Could you check a few things on this model? Use its own coordinates, in mm. Coordinates: 2 decimals unless noted, no trailing zeros. Loops run counter-clockwise (first coordinate to the right, second up) from the corner with the lowest first, then second, coordinate; pieces in that order, holes last. Notation, with made-up numbers: (57.25, 55.25) - (90.25, 55.25) arc R29 ccw to (90.25, 83.25) - close; hole circle Ø10 at (-29.75, 55). An arc over 180 degrees is marked (long way). One line per question, with ' | ' between items. Start each with the question number.
1. Please list where these lines run through material, in increasing order: L1, parallel to Y at x = -16.5, z = 0.25; L2, parallel to X at y = 40.5, z = 0; L3, parallel to Y at x = -9.5, z = 0.45. Write a range as [from, to].
2. I want a section at A-A, the plane x = 0. Write out the boundary of the cut face in (y, z), then the cut area to 3 significant figures.
3. I want a section at C-C, the plane z = -0.1. Count the separate pieces of the cut face and the enclosed holes in it, then the cut area to 3 significant figures.
4. I'm going to push a flat-ended pin straight in: P1, Ø0.5, axis at x = -40.5, z = -0.5, coming from the +Y side. Where does the tip first touch, or does it pass through?
5. I want a section at B-B, the plane x = -16.5. Write out the boundary of the cut face in (y, z), then the cut area to 3 significant figures.
from build123d import *

# Parameters (mm, degrees)
SKETCH2_W            = 82.5
SKETCH2_H            = 99
SKETCH2_R            = 0.8
SKETCH2_R_2          = 1.5
PCB_EXTRUDE_DEPTH    = 0.8
CORNER_FILLETS_R     = 1
SKETCH4_R            = 1.5
SOLAR_HOLES_DEPTH    = 65.454421881
SOLAR_HOLE_FILLETS_R = 0.5
M2_CLEARANCE_HOLES_D = 2.6
SKETCH10_W           = 1.75
SKETCH10_H           = 2.6
CUT_EXTRUDE2_DEPTH   = 65.454421881


with BuildPart() as part:
    # Sketch2 → pcb extrude (new, symmetric)
    with BuildSketch(Plane.XY):
        Rectangle(SKETCH2_W, SKETCH2_H)
        with Locations((0, 46.95)):
            Circle(SKETCH2_R, mode=Mode.SUBTRACT)
        with Locations((-39.5, -30.25)):
            Circle(SKETCH2_R, mode=Mode.SUBTRACT)
        with Locations((-39.5, -0.25)):
            Circle(SKETCH2_R, mode=Mode.SUBTRACT)
        with Locations((-39.5, 29.75)):
            Circle(SKETCH2_R, mode=Mode.SUBTRACT)
        with Locations((39.5, -30.25)):
            Circle(SKETCH2_R, mode=Mode.SUBTRACT)
        with Locations((39.5, -0.25)):
            Circle(SKETCH2_R, mode=Mode.SUBTRACT)
        with Locations((39.5, 29.75)):
            Circle(SKETCH2_R, mode=Mode.SUBTRACT)
        with Locations((0, -46.95)):
            Circle(SKETCH2_R_2, mode=Mode.SUBTRACT)
        with Locations((-16.5, 20)):
            Circle(SKETCH2_R, mode=Mode.SUBTRACT)
        with Locations((16.5, 20)):
            Circle(SKETCH2_R, mode=Mode.SUBTRACT)
        with Locations((-16.5, -20)):
            Circle(SKETCH2_R, mode=Mode.SUBTRACT)
        with Locations((16.5, -20)):
            Circle(SKETCH2_R, mode=Mode.SUBTRACT)
    extrude(amount=PCB_EXTRUDE_DEPTH, both=True)

    # corner fillets
    corner_fillets_edges = [part.edges().sort_by_distance(p)[0] for p in [
        (41.25, 49.5, 0),
        (41.25, -49.5, 0),
        (-41.25, -49.5, 0),
        (-41.25, 49.5, 0),
    ]]
    fillet(corner_fillets_edges, radius=CORNER_FILLETS_R)

    # Sketch4 → solar holes (cut, through all)
    with BuildSketch(Plane.XY.offset(0.8)):
        with Locations((0, 46.95)):
            Circle(SKETCH4_R)
        with BuildLine():
            Line((6.7, 39.35), (-6.7, 39.35))
            Line((-6.7, 39.35), (-6.7, 46.65))
            Line((-6.7, 46.65), (-9.5, 46.65))
            ThreePointArc((-9.5, 46.65), (-10, 47.15), (-9.5, 47.65))
            Line((-9.5, 47.65), (-3, 47.65))
            Line((-3, 47.65), (-3, 45.05))
            Line((-3, 45.05), (3, 45.05))
            Line((3, 45.05), (3, 47.65))
            Line((3, 47.65), (9.5, 47.65))
            ThreePointArc((9.5, 47.65), (10, 47.15), (9.5, 46.65))
            Line((9.5, 46.65), (6.7, 46.65))
            Line((6.7, 46.65), (6.7, 39.35))
        make_face()
    extrude(amount=-SOLAR_HOLES_DEPTH, mode=Mode.SUBTRACT)

    # solar hole fillets
    solar_hole_fillets_edges = [part.edges().sort_by_distance(p)[0] for p in [
        (-6.7, 39.35, 0),
        (-6.7, 46.65, 0),
        (-3, 47.65, 0),
        (-3, 45.05, 0),
        (3, 45.05, 0),
        (3, 47.65, 0),
        (6.7, 46.65, 0),
        (6.7, 39.35, 0),
    ]]
    fillet(solar_hole_fillets_edges, radius=SOLAR_HOLE_FILLETS_R)

    # M2 Clearance Holes (through all)
    with Locations(Plane.XY.offset(0.8)):
        with Locations((-39.5, 29.75), (-39.5, -0.25), (-16.5, 20), (16.5, 20), (16.5, -20), (-16.5, -20), (39.5, 29.75), (39.5, -0.25), (39.5, -30.25), (-39.5, -30.25)):
            Hole(M2_CLEARANCE_HOLES_D / 2)

    # Sketch10 → Cut-Extrude2 (cut, through all)
    with BuildSketch(Plane.XY.offset(0.8)):
        with Locations((-40.375, 29.75)):
            Rectangle(SKETCH10_W, SKETCH10_H)
        with Locations((-40.375, -0.25)):
            Rectangle(SKETCH10_W, SKETCH10_H)
        with Locations((-40.375, -30.25)):
            Rectangle(SKETCH10_W, SKETCH10_H)
        with Locations((40.375, -30.25)):
            Rectangle(SKETCH10_W, SKETCH10_H)
        with Locations((40.375, -0.25)):
            Rectangle(SKETCH10_W, SKETCH10_H)
        with Locations((40.375, 29.75)):
            Rectangle(SKETCH10_W, SKETCH10_H)
    extrude(amount=-CUT_EXTRUDE2_DEPTH, mode=Mode.SUBTRACT)


solid = part.part
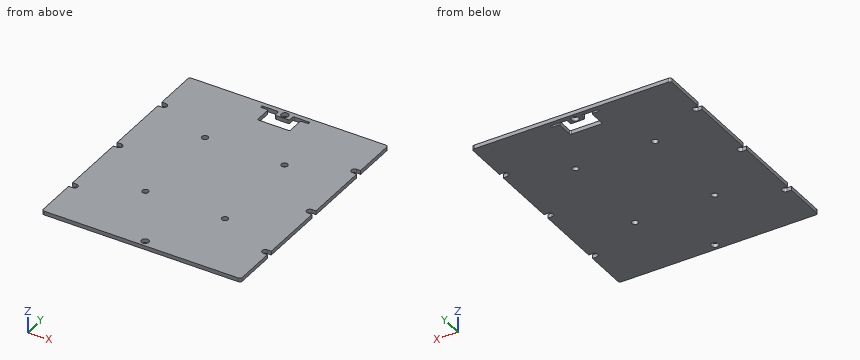
Results are:
1) L1: y = [-49.5, -21.3], [-18.7, 18.7], [21.3, 49.5] | L2: x = [-41.25, -6.7], [6.7, 41.25] | L3: y = [-49.5, 46.65], [47.65, 49.5]
2) outline: (-49.5, -0.8) - (-48.45, -0.8) - (-48.45, 0.8) - (-49.5, 0.8) - close; (-45.45, -0.8) - (39.35, -0.8) - (39.35, 0.8) - (-45.45, 0.8) - close; (45.05, -0.8) - (45.45, -0.8) - (45.45, 0.8) - (45.05, 0.8) - close; (48.45, -0.8) - (49.5, -0.8) - (49.5, 0.8) - (48.45, 0.8) - close | area: 140 mm2
3) separate pieces: 1 | enclosed holes: 7 | area: 7,990 mm2
4) P1: stops at y = 49.5
5) outline: (-49.5, -0.8) - (-21.3, -0.8) - (-21.3, 0.8) - (-49.5, 0.8) - close; (-18.7, -0.8) - (18.7, -0.8) - (18.7, 0.8) - (-18.7, 0.8) - close; (21.3, -0.8) - (49.5, -0.8) - (49.5, 0.8) - (21.3, 0.8) - close | area: 150 mm2
